CAD build for the part. Positions are in the model's coordinates, mm. A direction names the side the tool comes from. Coordinates: 2 decimals unless noted, no trailing zeros. Write each loop counter-clockwise with the first axis right and the second up, starting at its lowest first coordinate (ties: lowest second). Pieces come first, ordered by that corner, then holes. Notation, with made-up numbers: (17, 47.5) - (47, 47.5) arc R12 ccw to (47, 51.5) - close; hole circle Ø11 at (30, -20). An arc over 180 degrees is marked (long way). Answer in a Markdown table with one row per item. Add a question column.
Q1. Band-saw the part on A-A (x = -33). List the corners of the cut face in (y, z).
Q2. Band-saw the part on C-C (z = 13.5). List the corners of the cut face in (x, y), and give its area (3 significant figures).
Q3. Drill centre lines: line 1 along Y through (x, z) = (-11, 18.5); line 2 along X through (y, z) = (31, 18.5); line 3 along Z through (x, y) = (-50, 10.5). Where is each one in solid material? Low to high. Write a range as from..to.
Q4. Band-saw the part on B-B (y = 79). List the corners of the cut face in (x, z).
Q5. 3-axis set-ups, long thin cutter, end or side, ignore diameter. For faces 1 (the cylindrical face through (-148, 99, 18)), 2 (the flat face through (-76, 95, 15)): which of +Z, -Z, +X, -X, +Y, -Y reach the whole face in a straight line?
Q6. Pin check, flat tip, straight feed: pin 1 (1 mm diameter, centred on x = -72.5, y = 37, fed in from -Z). Stop position of the tip, or through.
Q7. Two-plate mould, pull along X, no slides. Class faces 3 (the flat face through (-76, 0, 17)), 4 (the flat face through (-145, 49, 15)), 5 (the cylindrical face through (-1, 98, 18)): +X half, -X half, draft (parallel to the pull), parting line (faces both ways), or undercut.
```python
from build123d import *

# Parameters (mm, degrees)
F0_W     = 140
F0_H     = 5
F0_H_2   = 90
F1_DEPTH = 35
F2_DEPTH = 31
F3_R     = 5


with BuildPart() as f1:
    # F0 (on Top) → F1 (new body)
    with BuildSketch(Plane.XY):
        Polygon((-145, 0), (0, 0), (0, 5), (-5, 5), (-145, 5), align=None)
        Polygon((-150, 0), (-145, 0), (-145, 5), (-145, 95), (-145, 100), (-150, 100), align=None)
        Polygon((-5, 5), (0, 5), (0, 100), (-5, 100), (-5, 95), align=None)
        with Locations((-75, 97.5)):
            Rectangle(F0_W, F0_H)
        with Locations((-75, 50)):
            Rectangle(F0_W, F0_H_2)
    extrude(amount=F1_DEPTH)

    # F0 (on Top) → F2 (cut)
    with BuildSketch(Plane.XY):
        with Locations((-75, 50)):
            Rectangle(F0_W, F0_H_2)
    extrude(amount=F2_DEPTH, mode=Mode.SUBTRACT)

    # F3
    f3_edges = [f1.edges().sort_by_distance(p)[0] for p in [
        (0, 0, 17.5),
        (0, 100, 17.5),
        (-150, 100, 17.5),
        (-150, 0, 17.5),
    ]]
    fillet(f3_edges, radius=F3_R)


solid = f1.part
```
Checked values:
| question | item | result |
|---|---|---|
| 1 | outline | (0, 0) - (5, 0) - (5, 31) - (95, 31) - (95, 0) - (100, 0) - (100, 35) - (0, 35) - close |
| 2 | outline | (-150, 5) arc R5 ccw to (-145, 0) - (-5, 0) arc R5 ccw to (0, 5) - (0, 95) arc R5 ccw to (-5, 100) - (-145, 100) arc R5 ccw to (-150, 95) - close; hole (-145, 5) - (-5, 5) - (-5, 95) - (-145, 95) - close |
| 2 | area | 2,380 mm² |
| 3 | line 1 | y = 0..5, 95..100 |
| 3 | line 2 | x = -150..-145, -5..0 |
| 3 | line 3 | z = 31..35 |
| 4 | outline | (-150, 0) - (-145, 0) - (-145, 31) - (-5, 31) - (-5, 0) - (0, 0) - (0, 35) - (-150, 35) - close |
| 5 | face 1 | +Z, -Z, -X, +Y |
| 5 | face 2 | -Z |
| 6 | pin 1 | stops at z = 31 |
| 7 | face 3 | draft |
| 7 | face 4 | undercut |
| 7 | face 5 | +X half |
